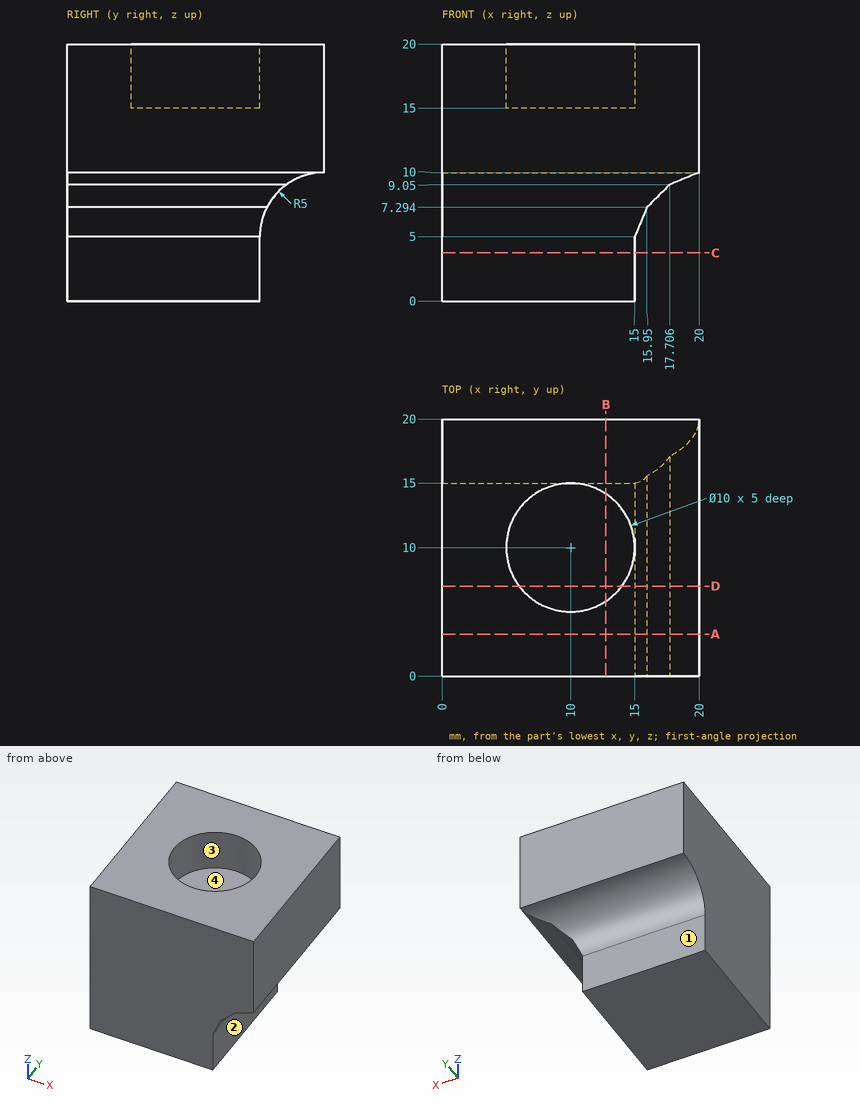
Verification items for this drawing (mm, ordinates from the low corner). Coordinates: 2 decimals unless noted, no trailing zeros. Order: outer loops, then holes, each group sorted by start corner. A loop starts at its lowest first (then second) coordinate and runs counter-clockwise, first axis right, second up. Notation, with made-up numbers: M 7,50 L 44,50 A23 cw 44,82 Z; hole C 74,20.5 d3. An arc over 180 degrees is marked long. One line per item, written item: value. Start each with the question number.
Item 1: Sectioned sample at C-C on z = 3.75. Record the cut outline in (x, y), then the cut area to 3 significant figures.
Item 2: Thickness scan on probe 1 along Y at (x, z) = (10, 18.4); probe 2 along X at (y, z) = (6, 5); probe 3 along Y at (x, z) = (13.75, 16). Record the ranges inside material, lowest first.
Item 3: Sectioned sample at D-D on y = 7. Record the cut outline in (x, z), then the cut area to 3 significant figures.
Item 4: Sectioned sample at A-A on y = 3.25. Record the cut outline in (x, z), then the cut area to 3 significant figures.
Item 5: Depth check by flat-ended pin: P1, Ø5.5, axis at x = 7.5, z = 2.5, coming from the +Y side; P2, Ø3, axis at x = 9, y = 12, coming from the +Z side; P3, Ø5.5, axis at y = 7, z = 2.5, coming from the +X side. Enter the tip coordinate at first touch or a pass-through.
Item 6: Sectioned sample at B-B on x = 12.75. Record the cut outline in (y, z), then the cut area to 3 significant figures.
Item 7: Mould release check, pull along Y, two halves, no side actions. Record for the marked faces 1, 2, 3 and 4: pulls with the +Y half, pulls with the -Y half, needs draft (parallel to the pull), parting line crosses it, or undercut.
Calculated:
1. outline: M 0,0 L 15,0 L 15,15 L 0,15 Z
1. area: 225 mm^2
2. probe 1: 0 to 5, 15 to 20
2. probe 2: 0 to 15
2. probe 3: 0 to 6.69, 13.31 to 20
3. outline: M 0,0 L 15,0 L 15,5 L 15.95,7.29 L 17.71,9.05 L 20,10 L 20,20 L 14,20 L 14,15 L 6,15 L 6,20 L 0,20 Z
3. area: 318 mm^2
4. outline: M 0,0 L 15,0 L 15,5 L 15.95,7.29 L 17.71,9.05 L 20,10 L 20,20 L 0,20 Z
4. area: 358 mm^2
5. P1: y = 15.01
5. P2: z = 15
5. P3: x = 15.1
6. outline: M 0,0 L 15,0 L 15,5 A5 cw 20,10 L 20,20 L 14.18,20 L 14.18,15 L 5.82,15 L 5.82,20 L 0,20 Z
6. area: 314 mm^2
7. face 1: pulls with the +Y half
7. face 2: needs draft
7. face 3: undercut
7. face 4: undercut
